Autodesk Fusion 360 part; units mm, degrees
sketch "main" plane through (0, 0, 0) normal (0, 0, 1) x (1, 0, 0)
  circle A0 centre (0, 0) radius 2.25
  line L0 (-3.5, 5) -> (3.5, 5)
  line L1 (5, 3.5) -> (5, -3.5)
  line L2 (3.5, -5) -> (-3.5, -5)
  line L3 (-5, -3.5) -> (-5, 3.5)
  line L4 (-5, 5) -> (5, -5) construction
  line L5 (5, 5) -> (-5, -5) construction
  arc A1 (-3.5, 5) -> (-5, 3.5) centre (-3.5, 3.5) ccw
  arc A2 (-5, -3.5) -> (-3.5, -5) centre (-3.5, -3.5) ccw
  arc A3 (3.5, -5) -> (5, -3.5) centre (3.5, -3.5) ccw
  arc A4 (5, 3.5) -> (3.5, 5) centre (3.5, 3.5) ccw
  circle A5 centre (0, 0) radius 20
  line L6 (0, 5) -> (0, 15) construction
  line L7 (0, -15) -> (0, -5) construction
  circle A6 centre (0, 15) radius 1.75
  line L8 (3.465, 15) -> (1.7325, 18.0008)
  line L9 (1.7325, 18.0008) -> (-1.7325, 18.0008)
  line L10 (-1.7325, 18.0008) -> (-3.465, 15)
  line L11 (-3.465, 15) -> (-1.7325, 11.9992)
  line L12 (-1.7325, 11.9992) -> (1.7325, 11.9992)
  line L13 (1.7325, 11.9992) -> (3.465, 15)
  circle A7 centre (0, -15) radius 1.75
  line L14 (3.465, -15) -> (1.7325, -11.9992)
  line L15 (1.7325, -11.9992) -> (-1.7325, -11.9992)
  line L16 (-1.7325, -11.9992) -> (-3.465, -15)
  line L17 (-3.465, -15) -> (-1.7325, -18.0008)
  line L18 (-1.7325, -18.0008) -> (1.7325, -18.0008)
  line L19 (1.7325, -18.0008) -> (3.465, -15)
  circle A8 centre (0, 0) radius 55
  spline S0 degree 5 poles (-5.0305, 19.357) (-4.9656, 19.5382) (-4.8376, 19.914) (-4.6506, 20.5186) (-4.4115, 21.4066) (-4.1299, 22.6499) (-3.8662, 24.0155) (-3.6214, 25.4797) (-3.3969, 26.9998) (-3.1947, 28.5187) (-3.017, 29.9798) (-2.8658, 31.3385) (-2.7432, 32.5744) (-2.6507, 33.707) (-2.5895, 34.7948) (-2.5603, 35.9102) (-2.5641, 37.1227) (-2.6015, 38.476) (-2.6738, 39.9752) (-2.7821, 41.5999) (-2.9274, 43.3124) (-3.1108, 45.0674) (-3.3328, 46.8208) (-3.5937, 48.5404) (-3.8934, 50.2058) (-4.2314, 51.805) (-4.5322, 53.0272) (-4.7748, 53.9111) (-4.944, 54.4858) (-5.0305, 54.7695) knots 0 0 0 0 0 0 0.04 0.08 0.12 0.16 0.2 0.24 0.28 0.32 0.36 0.4 0.44 0.48 0.52 0.56 0.6 0.64 0.68 0.72 0.76 0.8 0.84 0.88 0.92 0.96 1 1 1 1 1 1
  spline S1 degree 5 poles (5.0305, 19.357) (4.9656, 19.5382) (4.8376, 19.914) (4.6506, 20.5186) (4.4115, 21.4066) (4.1299, 22.6499) (3.8662, 24.0155) (3.6214, 25.4797) (3.3969, 26.9998) (3.1947, 28.5187) (3.017, 29.9798) (2.8658, 31.3385) (2.7432, 32.5744) (2.6507, 33.707) (2.5895, 34.7948) (2.5603, 35.9102) (2.5641, 37.1227) (2.6015, 38.476) (2.6738, 39.9752) (2.7821, 41.5999) (2.9274, 43.3124) (3.1108, 45.0674) (3.3328, 46.8208) (3.5937, 48.5404) (3.8934, 50.2058) (4.2314, 51.805) (4.5322, 53.0272) (4.7748, 53.9111) (4.944, 54.4858) (5.0305, 54.7695) knots 0 0 0 0 0 0 0.04 0.08 0.12 0.16 0.2 0.24 0.28 0.32 0.36 0.4 0.44 0.48 0.52 0.56 0.6 0.64 0.68 0.72 0.76 0.8 0.84 0.88 0.92 0.96 1 1 1 1 1 1
  line L20 (-5.983, 16.697) -> (-4.078, 22.017)
  line L21 (-4.0792, 51.649) -> (-5.9817, 57.8899)
  line L22 (5.983, 16.697) -> (4.078, 22.017)
  line L23 (4.0792, 51.649) -> (5.9817, 57.8899)
  circle A9 centre (0, 0) radius 60
  point P0 (0, 15)
  point P1 (0, -15)
  point P2 (-3.7631, 24.6573)
  point P3 (-2.8027, 31.9975)
  point P4 (-2.5682, 36.8246)
  point P5 (-3.1758, 45.5337)
  point P6 (3.7631, 24.6573)
  point P7 (2.8027, 31.9975)
  point P8 (2.5682, 36.8246)
  point P9 (3.1758, 45.5337)
  dimension "d1" = 4.5
  dimension "d2" = 10
  dimension "d3" = 10
  dimension "d4" = 1.5
  dimension "d5" = 40
  dimension "d6" = 10
  dimension "d7" = 10
  dimension "d8" = 3.5
  dimension "d9" = 3.465
  dimension "d10" = 3.5
  dimension "d11" = 3.465
  dimension "d12" = 110
  dimension "d23" = 120
extrude "Extrude1" add sketch "main" along normal blind 7.5 contours A5 A8 S0 S1 picked at (-13.7602, 33.1549) makes body 1
pattern_circular "C-Pattern1" count 4 over 360 about axis through (0, 0, 1.75) along (0, 0, 1) of "Extrude1" makes body 2 makes body 3 makes body 4
extrude "Extrude2" add sketch "main" along normal blind 7.5 contours A5 bodies 1 2 3 4
extrude "Extrude3" add sketch "main" along normal blind 17.5 contours L0 L1 L2 L3 A1 A2 A3 A4 bodies 1
extrude "Extrude4" add sketch "main" along normal blind 4.5 contours L8 L9 L10 L11 L12 L13 | L14 L15 L16 L17 L18 L19 bodies 1
extrude "Extrude5" add sketch "main" along normal blind 15 contours A9 bodies 1
fillet "Fillet1" radius 2 2 edges at (-55.9396, -21.6969, 0) (-55.9396, -21.6969, 15) on bodies 1
equation "d9 = ( 6.93 / 2 ) * 1 mm"
equation "d11 = ( 6.93 / 2 ) * 1 mm"
equation "d21 = 7.50 mm - 3 mm"
Could you check a few things on this model? Use its own coordinates, in mm. A direction names the side the tool comes from. Round coordinates to 2 decimals unless told otherwise and drop trailing zeros. Loops run counter-clockwise (first coordinate to the right, second up) from the corner with the lowest first, then second, coordinate; pieces in that order, holes last. Notation, with made-up numbers: M 12.25,68 L 44.25,68 A27 cw 44.25,88 Z; hole C 29.25,13.25 d2. An arc over 180 degrees is marked long. Answer as CSV lines item,"result".
1) Which directions (+Z, -Z, +X, -X, +Y, -Y) give clear straight access to the entire face, cutting with the end or side of a thin tool? Please do faces 4 (the cylindrical face through (-0.228, -16.735, 2.218)), 5 (the flat face through (1.5, -13.6, 4.5)).
From the geometry:
face 4,"+Z, -Z"
face 5,"+Z"
2) If I drill on probe 1 along Y at (x, z) = (0, 1.85); probe 2 along Y at (x, z) = (0, 13); probe 3 along X at (y, z) = (38, 9), over which ranges is the centre line in solid material (lowest first)?
From the geometry:
probe 1,"-59.99 to -16.75, -13.25 to -2.25, 2.25 to 13.25, 16.75 to 59.99"
probe 2,"-60 to -55, -5 to -2.25, 2.25 to 5, 55 to 60"
probe 3,"-46.43 to -39.76, 39.76 to 46.43"
3) We'd pull the mould along X, two halves only. Please class faces 1 (the flat face through (2.6, -13.5, 6)), 2 (the flat face through (-2.6, 16.5, 6)), 3 (the flat face through (51, -21, 15)): released by +X, released by -X, zero draft, split by the parting line, or undercut.
From the geometry:
face 1,"undercut"
face 2,"undercut"
face 3,"zero draft"
4) For pin 1 Ø5.5 at (x, z) = (-0.5, 11) entering from -Y; pin 2 Ø2.5 at (x, z) = (0, 5.5) entering from +Y; pin 3 Ø3 at (x, y) = (1.5, 15) entering from +Z, each with a flat end and sliding along its axis, tell me the tip position at first contact or that it passes through.
From the geometry:
pin 1,"y = -60"
pin 2,"y = 60"
pin 3,"z = 4.5"
5) Imagine slicing it at A-A on y = 0. List the corners of the cut face in (x, z) for me, and give its area (3 significant figures).
From the geometry:
outline,"M -60,2 A2 ccw -58,0 L -2.25,0 L -2.25,17.5 L -5,17.5 L -5,7.5 L -55,7.5 L -55,15 L -58,15 A2 ccw -60,13 Z; M 2.25,0 L 58,0 A2 ccw 60,2 L 60,13 A2 ccw 58,15 L 55,15 L 55,7.5 L 5,7.5 L 5,17.5 L 2.25,17.5 Z"
area,"993 mm^2"
6) Imagine slicing it at B-B on x = 0. Count the separate pieces of the cut face and the enclosed holes in it, and give its area (3 significant figures).
From the geometry:
separate pieces,"4"
enclosed holes,"0"
area,"925 mm^2"
